The model under review builds one solid part; all positions refer to its coordinate system, in mm. Face numbers are marked on the shaded views. A direction names the side the tool comes from. Round coordinates to 2 decimals unless told otherwise and drop trailing zeros. Order: outer loops, then holes, each group sorted by start corner. A loop starts at its lowest first (then second) coordinate and runs counter-clockwise, first axis right, second up.
1) Consider section A-A (z = 0). Give the boundary of the cut face in (x, y).
2) To check wall thickness, follow L1, parallel to Z at x = 0, y = 3.25; L2, parallel to X at y = -1.5, z = 0.7; L3, parallel to X at y = 0, z = -0.85. State the ranges of each line that lie inside material, in increasing order.
3) Consider section C-C (z = 1.05). Give the boundary of the cut face in (x, y), then the cut area to 3 significant figures.
4) Consider section B-B (y = -0.25). Give the boundary of the cut face in (x, z).
5) Machinability: for the marked faces 1, 2 and 3, which of the approach directions +Z, -Z, +X, -X, +Y, -Y give a long, thin tool a straight path to every point of the face, cutting with its end or side? Answer none if there is none.
6) Consider section D-D (y = 3). Give the boundary of the cut face in (x, z), then the cut area to 3 significant figures.
7) Clearance check with a flat-ended pin moving along its axis: P1, Ø3, axis at x = 16, y = 3.5, coming from the -Z side. State where the tip first meets the part, or that it passes through.
8) Mouldability with a two-part tool opening along X and no side actions: class the marked faces 4, 5 and 6 as pulls with the +X half, pulls with the -X half, needs draft (parallel to the pull), parting line crosses it, or undercut.
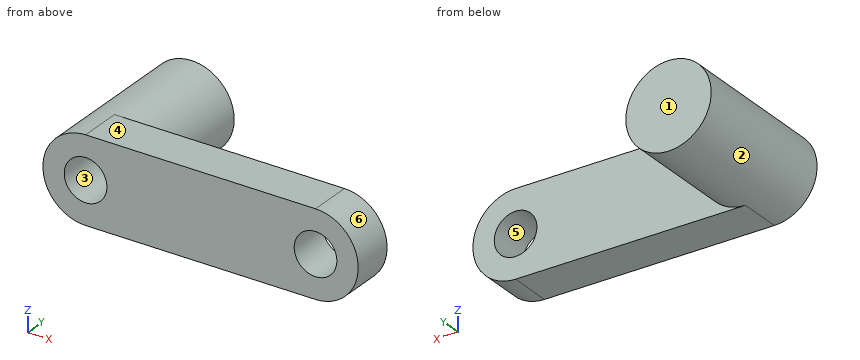
from build123d import *

# Parameters (mm, degrees)
SKETCH1_R           = 3
BOSS_EXTRUDE1_DEPTH = 9
SKETCH4_R           = 3
BOSS_EXTRUDE3_DEPTH = 2
SKETCH6_R           = 1.5
BOSS_EXTRUDE4_DEPTH = 3
SKETCH7_R           = 1.5
CUT_EXTRUDE3_DEPTH  = 10


with BuildPart() as part:
    # Sketch1 → Boss-Extrude1 (new body)
    with BuildSketch(Plane(origin=(0, 0, 0), x_dir=(1, 0, 0), z_dir=(0, 1, 0))):
        Circle(SKETCH1_R)
    extrude(amount=BOSS_EXTRUDE1_DEPTH)

    # Sketch4 → Boss-Extrude3 (add)
    with BuildSketch(Plane.XZ):
        Circle(SKETCH4_R)
    extrude(amount=BOSS_EXTRUDE3_DEPTH)

    # Sketch6 → Boss-Extrude4 (add)
    with BuildSketch(Plane.XZ.offset(2)):
        with BuildLine():
            Line((16.163723902, 3), (0, 3))
            ThreePointArc((0, 3), (2.121320344, 2.121320344), (3, 0))
            ThreePointArc((3, 0), (2.121320344, -2.121320344), (0, -3))
            Line((0, -3), (16.163723902, -3))
            ThreePointArc((16.163723902, -3), (19.163723902, 0), (16.163723902, 3))
        make_face()
        with Locations((16.163723902, 0)):
            Circle(SKETCH6_R, mode=Mode.SUBTRACT)
    extrude(amount=-BOSS_EXTRUDE4_DEPTH)

    # Sketch7 → Cut-Extrude3 (cut)
    with BuildSketch(Plane.XZ.offset(2)):
        Circle(SKETCH7_R)
    extrude(amount=-CUT_EXTRUDE3_DEPTH, mode=Mode.SUBTRACT)


solid = part.part
Answer below:
1. outline: (-3, -2) - (-1.5, -2) - (-1.5, 8) - (1.5, 8) - (1.5, -2) - (14.66, -2) - (14.66, 1) - (3, 1) - (3, 9) - (-3, 9) - close; (17.66, -2) - (19.16, -2) - (19.16, 1) - (17.66, 1) - close
2. L1: z = -3 to -1.5, 1.5 to 3
2. L2: x = -2.92 to -1.33, 1.33 to 14.84, 17.49 to 19.08
2. L3: x = -2.88 to -1.24, 1.24 to 14.93, 17.4 to 19.04
3. outline: (-2.81, -2) - (-1.07, -2) - (-1.07, 8) - (1.07, 8) - (1.07, -2) - (15.09, -2) - (15.09, 1) - (2.81, 1) - (2.81, 9) - (-2.81, 9) - close; (17.23, -2) - (18.97, -2) - (18.97, 1) - (17.23, 1) - close
3. area: 82.5 mm2
4. outline: (0, -3) - (16.16, -3) arc R3 ccw to (16.16, 3) - (0, 3) arc R3 ccw to start; hole circle Ø3 at (0, 0); hole circle Ø3 at (16.16, 0)
5. face 1: +Z, -Z, +X, -X, +Y
5. face 2: +Y
5. face 3: -Y
6. outline: circle Ø6 at (0, 0); hole circle Ø3 at (0, 0)
6. area: 21.2 mm2
7. P1: passes through
8. face 4: needs draft
8. face 5: undercut
8. face 6: pulls with the +X half
